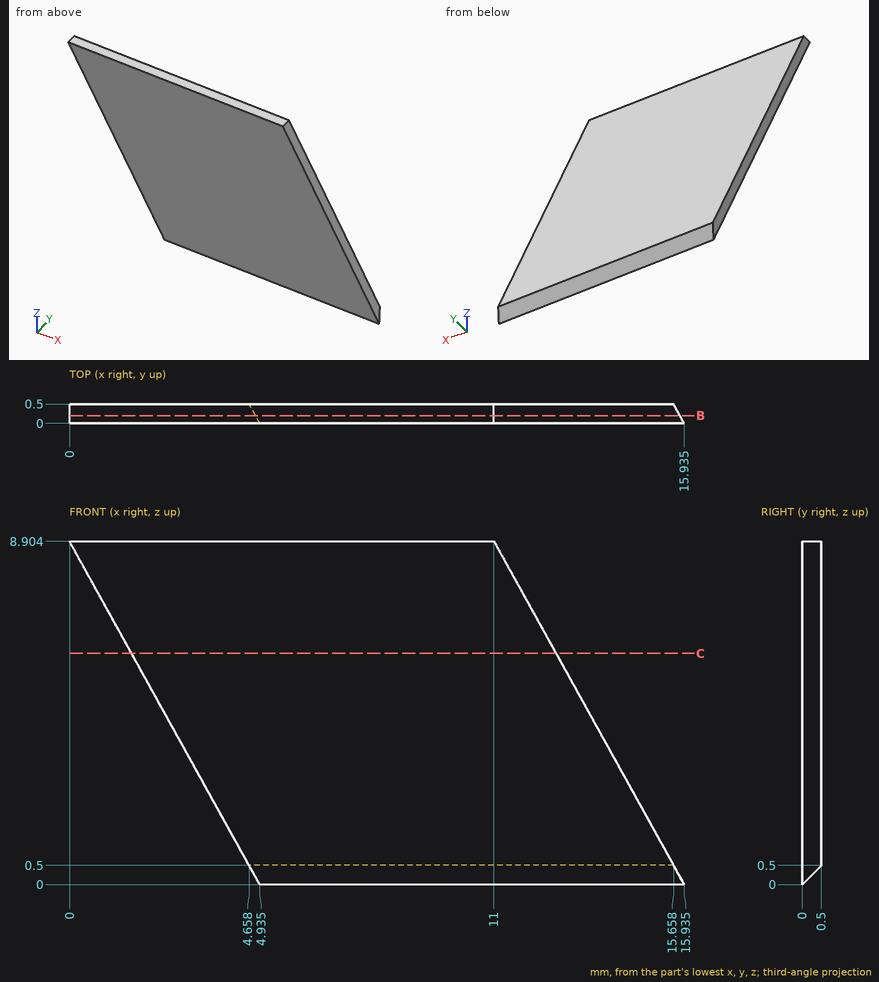
Source: three-view drawing plus pictorial views. Frame: mm from the lowest corner of the part. Round coordinates to 2 decimals unless told otherwise and drop trailing zeros. Write each loop counter-clockwise with the first axis right and the second up, starting at its lowest first coordinate (ties: lowest second). Pieces come first, ordered by that corner, then holes. Notation, with made-up numbers: (78, 78) -> (115, 78) arc R22 ccw to (115, 88) -> close; hole circle Ø3 at (50.5, 26.5). An arc over 180 degrees is marked (long way). Return JSON: item names as keys, results as strings.
Q1. Ray query, line 1 (X direction, y = 0.25, z = 7) (1 decimal); line 2 (Z direction, x = 11.75, y = 0.15); line 3 (X direction, y = 0.4, z = 1.75) (1 decimal). Return the intervals inside material, ascending.
From the geometry:
{"line 1": "1.1 to 12.1", "line 2": "0.15 to 7.55", "line 3": "4 to 15"}
Q2. Section B-B on y = 0.2. Return the cut outline in (x, z) (1 decimal).
From the geometry:
{"outline": "(0, 8.9) -> (4.8, 0.2) -> (15.8, 0.2) -> (11, 8.9) -> close"}
Q3. Section C-C on z = 6. Return the cut outline in (x, y).
From the geometry:
{"outline": "(1.61, 0) -> (12.61, 0) -> (12.61, 0.5) -> (1.61, 0.5) -> close"}
